Geometry check sheet. Reference: the model listing, model coordinates, mm. A direction names the side the tool comes from. Coordinates: 2 decimals unless noted, no trailing zeros. Loops run counter-clockwise (first coordinate to the right, second up) from the corner with the lowest first, then second, coordinate; pieces in that order, holes last.
from build123d import *

# Parameters (mm, degrees)
BOSS_EXTRUDE1_DEPTH = 609.6
SKETCH2_R           = 4
CUT_EXTRUDE1_DEPTH  = 611.956962478
SKETCH3_R           = 4
CUT_EXTRUDE2_DEPTH  = 611.956962478


with BuildPart() as part:
    # Sketch1 → Boss-Extrude1 (new body)
    with BuildSketch(Plane.XY):
        Polygon((0, 0), (0, 30), (2.5, 30), (2.5, 2.5), (30, 2.5), (30, 0), align=None)
    extrude(amount=BOSS_EXTRUDE1_DEPTH)

    # Sketch2 → Cut-Extrude1 (cut, through all)
    with BuildSketch(Plane(origin=(2.5, 0, 0), x_dir=(0, 0, -1), z_dir=(1, 0, 0))):
        with Locations(Location((-594.6, 15, 0), (0, 0, 90))):
            Circle(SKETCH2_R)
        with Locations(Location((-15, 15, 0), (0, 0, 270))):
            Circle(SKETCH2_R)
        with Locations(Location((-431.3434763, 15, 0), (0, 0, 90))):
            Circle(SKETCH2_R)
        with Locations(Location((-178.2565237, 15, 0), (0, 0, 270))):
            Circle(SKETCH2_R)
    extrude(amount=-CUT_EXTRUDE1_DEPTH, mode=Mode.SUBTRACT)

    # Sketch3 → Cut-Extrude2 (cut, through all)
    with BuildSketch(Plane(origin=(0, 2.5, 0), x_dir=(1, 0, 0), z_dir=(0, 1, 0))):
        with Locations(Location((15, -12.5, 0), (0, 0, 180))):
            Circle(SKETCH3_R)
        with Locations(Location((15, -597.1, 0), (0, 0, 180))):
            Circle(SKETCH3_R)
    extrude(amount=-CUT_EXTRUDE2_DEPTH, mode=Mode.SUBTRACT)


solid = part.part
(1) Access from +Z, -Z, +X, -X, +Y, -Y to the whole of each face (thin tool, end or side, straight path). Record for faces 4 (the flat face through (16, 2.5, 301)), 5 (the flat face through (15, 0, 301)).
Findings:
face 4: +Z, -Z, +X, +Y
face 5: +Z, -Z, +X, -X, -Y
(2) Sectioned sample at B-B on y = 25. Record the cut outline in (x, z).
Findings:
outline: (0, 0) - (2.5, 0) - (2.5, 609.6) - (0, 609.6) - close
(3) Draft check along Z on faces 1 (the flat face through (8, 2, 0)), 2 (the flat face through (8, 2, 609.6)), 3 (the flat face through (2.5, 16, 301)). Enter one of: +Z half, -Z half, draft (parallel to the pull), parting line (faces both ways), or undercut.
Findings:
face 1: -Z half
face 2: +Z half
face 3: draft
(4) Gauge pin test, flat ends, axial feed: pin 1 Ø10 at (x, z) = (13, 387) entering from +Y; pin 2 Ø1.5 at (y, z) = (12.5, 339) entering from +X. Record the tip position at first contact, or that the pin passes through.
Findings:
pin 1: stops at y = 2.5
pin 2: stops at x = 2.5
(5) Scan lines: L1, parallel to Z at x = 1.5, y = 15; L2, parallel to Y at x = 1.75, z = 594.6; L3, parallel to Z at x = 15, y = 1.55. Record each from-to range of solid material in increasing order.
Findings:
L1: z = 0 to 11, 19 to 174.26, 182.26 to 427.34, 435.34 to 590.6, 598.6 to 609.6
L2: y = 0 to 11, 19 to 30
L3: z = 0 to 8.5, 16.5 to 593.1, 601.1 to 609.6
(6) Sectioned sample at A-A on z = 394. Record the cut outline in (x, y), and give its area (3 significant figures).
Findings:
outline: (0, 0) - (30, 0) - (30, 2.5) - (2.5, 2.5) - (2.5, 30) - (0, 30) - close
area: 144 mm2
